```python
from build123d import *

# Parameters (mm, degrees)
SKETCH_1_W          = 250
SKETCH_1_H          = 250
EXTRUDE_1_DEPTH     = 36
CUT_EXTRUDE_1_REACH = 357.381
SKETCH_2_R          = 30
SKETCH_3_R          = 38.5
CUT_EXTRUDE_2_DEPTH = 5.5
SKETCH_4_W          = 25
SKETCH_4_H          = 230
EXTRUDE_2_DEPTH     = 200
CUT_EXTRUDE_3_REACH = 399.146


with BuildPart() as part:
    # 草图1 → 凸台-拉伸1 (new body)
    with BuildSketch(Plane(origin=(0, 0, 0), x_dir=(1, 0, 0), z_dir=(0, 1, 0))):
        with Locations((125, -125)):
            Rectangle(SKETCH_1_W, SKETCH_1_H)
    extrude(amount=EXTRUDE_1_DEPTH)

    # 草图2 → 切除-拉伸1 (cut, up to next)
    with BuildSketch(Plane(origin=(0, 36, 0), x_dir=(1, 0, 0), z_dir=(0, 1, 0)), mode=Mode.PRIVATE) as cut_extrude_1_sk1:
        with Locations(Location((125, -170, 0), (0, 0, 270))):
            Circle(SKETCH_2_R)
    cut_extrude_1_tool1 = extrude(cut_extrude_1_sk1.sketch, amount=-CUT_EXTRUDE_1_REACH, mode=Mode.PRIVATE) & part.part
    add(cut_extrude_1_tool1.solids().sort_by_distance((125, 36, 170))[0], mode=Mode.SUBTRACT)

    # 草图3 → 切除-拉伸2 (cut)
    with BuildSketch(Plane(origin=(0, 36, 0), x_dir=(1, 0, 0), z_dir=(0, 1, 0))):
        with Locations(Location((125, -170, 0), (0, 0, 270))):
            Circle(SKETCH_3_R)
    extrude(amount=-CUT_EXTRUDE_2_DEPTH, mode=Mode.SUBTRACT)

    # 草图4 → 凸台-拉伸2 (add)
    with BuildSketch(Plane.XZ):
        with Locations((27.5, 115)):
            Rectangle(SKETCH_4_W, SKETCH_4_H)
    extrude_2 = extrude(amount=EXTRUDE_2_DEPTH)

    # 草图5 → 切除-拉伸3 (cut, up to next)
    with BuildSketch(Plane.ZY.offset(-15), mode=Mode.PRIVATE) as cut_extrude_3_sk1:
        Polygon((30, -200), (230, -30), (230, -200), align=None)
    cut_extrude_3_tool1 = extrude(cut_extrude_3_sk1.sketch, amount=-CUT_EXTRUDE_3_REACH, mode=Mode.PRIVATE) & part.part
    cut_extrude_3 = cut_extrude_3_tool1.solids().sort_by_distance((15, -143.333333, 163.333333))[0]
    add(cut_extrude_3, mode=Mode.SUBTRACT)

    # 镜向1: 凸台-拉伸2, 切除-拉伸3 across plane
    add(extrude_2.mirror(Plane(origin=(125, 0, 0), x_dir=(0, 0, 1), z_dir=(1, 0, 0))))
    add(cut_extrude_3.mirror(Plane(origin=(125, 0, 0), x_dir=(0, 0, 1), z_dir=(1, 0, 0))), mode=Mode.SUBTRACT)


solid = part.part
```
Model file for the job. Use its own axes, mm. A direction names the side the tool comes from. Give positions to 0.01 mm unless a question says otherwise; leave off trailing zeros. Write each loop counter-clockwise with the first axis right and the second up, starting at its lowest first coordinate (ties: lowest second). Pieces come first, ordered by that corner, then holes. Notation, with made-up numbers: (26, 50) - (84, 50) arc R7 cw to (84, 54) - close; hole circle Ø11 at (11.25, 21). An arc over 180 degrees is marked (long way). One line per question, with ' | ' between items. Start each with the question number.
(1) Slice it at D-D on y = -137. Write the cut outline in (x, z), plus the area to 3 significant figures.
(2) Slice it at B-B on x = 125. Write the cut outline in (y, z), plus the area to 3 significant figures.
(3) Two-plate mould, pull along Z, no slides. Class faces 6 (the face through (27, -15, 230)), 7 (the face through (105, 30.5, 193)), 8 (the face through (40, -76, 88)): +Z half, -Z half, draft (parallel to the pull), parting line (faces both ways), or undercut.
(4) Slice it at C-C on y = -4. Write the cut outline in (x, z).
(5) Pin check, flat tips, straight feed: P1, Ø6, axis at x = 55.5, z = 182, coming from the -Y side; P2, Ø4, axis at x = 225, y = -123.5, coming from the +Z side; P3, Ø20, axis at x = 219, y = -21, coming from the +Z side. Stop position of each tip, or through.
(6) 3-axis set-ups, long thin cutter, end or side, ignore diameter. For faces 1 (the face through (223, -15, 230)), 2 (the face through (15, -76, 88)), 3 (the face through (235, -76, 88)), 4 (the face through (87.416, 33.288, 161.654)), 5 (the face through (210, -76, 88)): which of +Z, -Z, +X, -X, +Y, -Y reach the whole face in a straight line?
(7) Slice it at A-A on z = 170. Write the cut outline in (x, y), plus the area to 3 significant figures.
(8) Wall check: line 1 along X through (y, z) = (-112.5, 130); line 2 along X through (y, z) = (33.8, 170); line 3 along Y through (x, z) = (89, 167). Give the ranges that are in metal, low to high. Write a range as from..to.
Results below:
1) outline: (15, 0) - (40, 0) - (40, 104.12) - (15, 104.12) - close; (210, 0) - (235, 0) - (235, 104.12) - (210, 104.12) - close | area: 5,210 mm^2
2) outline: (0, 0) - (36, 0) - (36, 131.5) - (30.5, 131.5) - (30.5, 140) - (0, 140) - close; (0, 200) - (30.5, 200) - (30.5, 208.5) - (36, 208.5) - (36, 250) - (0, 250) - close | area: 6,750 mm^2
3) face 6: +Z half | face 7: undercut | face 8: draft
4) outline: (15, 0) - (40, 0) - (40, 230) - (15, 230) - close; (210, 0) - (235, 0) - (235, 230) - (210, 230) - close
5) P1: y = 0 | P2: z = 122.35 | P3: z = 230
6) face 1: +Z, +X, -X, -Y | face 2: +Z, -Z, -X, -Y | face 3: +Z, -Z, +X, -Y | face 4: +Y | face 5: +Z, -Z, -Y
7) outline: (0, 0) - (15, 0) - (15, -81) - (40, -81) - (40, 0) - (95, 0) - (95, 30.5) - (86.5, 30.5) - (86.5, 36) - (0, 36) - close; (155, 0) - (210, 0) - (210, -81) - (235, -81) - (235, 0) - (250, 0) - (250, 36) - (163.5, 36) - (163.5, 30.5) - (155, 30.5) - close | area: 10,800 mm^2
8) line 1: 15..40, 210..235 | line 2: 0..86.5, 163.5..250 | line 3: 0..30.5
